```python
from build123d import *

# Parameters (mm, degrees)
ESQUISSE1_R             = 1
BOSS_EXTRU_1_DEPTH      = 6
ESQUISSE2_R             = 10
ESQUISSE2_R_2           = 2
ESQUISSE2_R_3           = 1.4
ESQUISSE2_R_4           = 1.5
ESQUISSE2_W             = 8
ESQUISSE2_H             = 55
ESQUISSE2_W_2           = 44
ESQUISSE2_W_3           = 40
ESQUISSE2_H_2           = 80
ENL_V_MAT_EXTRU_1_DEPTH = 6
ESQUISSE3_W             = 6
ESQUISSE3_H             = 10
ESQUISSE3_W_2           = 10
ESQUISSE3_H_2           = 6
ESQUISSE3_W_3           = 15
ENL_V_MAT_EXTRU_2_DEPTH = 6
ESQUISSE4_R             = 1.5
ENL_V_MAT_EXTRU_3_DEPTH = 6
ESQUISSE5_W             = 10
ESQUISSE5_H             = 6
ESQUISSE5_W_2           = 20
ENL_V_MAT_EXTRU_4_DEPTH = 6
ESQUISSE6_R             = 1.65
ESQUISSE6_R_2           = 1.5
ESQUISSE6_R_3           = 2
ENL_V_MAT_EXTRU_5_DEPTH = 6


with BuildPart() as part:
    # Esquisse1 → Boss.-Extru.1 (new body)
    with BuildSketch(Plane.XY):
        Polygon((-165, 96.73), (165, 96.73), (165, -18.27), (123, -109.022410436), (-123, -109.022410436), (-165, -18.27), align=None)
        with Locations((-23.6, -89.522410436)):
            Circle(ESQUISSE1_R, mode=Mode.SUBTRACT)
        with Locations((-23.6, -73.522410436)):
            Circle(ESQUISSE1_R, mode=Mode.SUBTRACT)
        with Locations((-39.6, -89.522410436)):
            Circle(ESQUISSE1_R, mode=Mode.SUBTRACT)
        with Locations((-39.6, -73.522410436)):
            Circle(ESQUISSE1_R, mode=Mode.SUBTRACT)
    extrude(amount=BOSS_EXTRU_1_DEPTH)

    # Esquisse2 → Enlèv. mat.-Extru.1 (cut)
    with BuildSketch(Plane.XY.offset(6)):
        with Locations((140, 76.73)):
            Circle(ESQUISSE2_R)
        with Locations((108, -89.022410436)):
            Circle(ESQUISSE2_R)
        with Locations((-140, 76.73)):
            Circle(ESQUISSE2_R)
        with Locations((-108, -89.022410436)):
            Circle(ESQUISSE2_R)
        with Locations((161, -16.022410436)):
            Circle(ESQUISSE2_R_2)
        with Locations((119, -105.022410436)):
            Circle(ESQUISSE2_R_2)
        with Locations((161, 92.73)):
            Circle(ESQUISSE2_R_2)
        with Locations((-161, 92.73)):
            Circle(ESQUISSE2_R_2)
        with Locations((-161, -16.022410436)):
            Circle(ESQUISSE2_R_2)
        with Locations((-119, -105.022410436)):
            Circle(ESQUISSE2_R_2)
        with Locations((125.27, 76.73)):
            Circle(ESQUISSE2_R_3)
        with Locations((110.27, 76.73)):
            Circle(ESQUISSE2_R_3)
        with Locations((114.7893454, -75.950391119)):
            Circle(ESQUISSE2_R_4)
        with Locations((121.703139086, -62.638762485)):
            Circle(ESQUISSE2_R_4)
        with Locations((-110.27, 76.73)):
            Circle(ESQUISSE2_R_3)
        with Locations((-125.27, 76.73)):
            Circle(ESQUISSE2_R_3)
        with Locations((-121.703139086, -62.638762485)):
            Circle(ESQUISSE2_R_4)
        with Locations((-114.7893454, -75.950391119)):
            Circle(ESQUISSE2_R_4)
        with Locations((-154, 28.477589564)):
            Rectangle(ESQUISSE2_W, ESQUISSE2_H)
        with Locations((-108, 28.477589564)):
            Rectangle(ESQUISSE2_W_2, ESQUISSE2_H)
        with Locations((108, 28.477589564)):
            Rectangle(ESQUISSE2_W_2, ESQUISSE2_H)
        with Locations((154, 28.477589564)):
            Rectangle(ESQUISSE2_W, ESQUISSE2_H)
        with Locations((69, -69.022410436)):
            Rectangle(ESQUISSE2_W_3, ESQUISSE2_H_2)
        with Locations((-69, -69.022410436)):
            Rectangle(ESQUISSE2_W_3, ESQUISSE2_H_2)
    extrude(amount=-ENL_V_MAT_EXTRU_1_DEPTH, mode=Mode.SUBTRACT)

    # Esquisse3 → Enlèv. mat.-Extru.2 (cut)
    with BuildSketch(Plane(origin=(0, 0, 0), x_dir=(-1, 0, 0), z_dir=(0, 0, -1))):
        with Locations((162, 1.73)):
            Rectangle(ESQUISSE3_W, ESQUISSE3_H)
        with Locations((162, 73.852589564)):
            Rectangle(ESQUISSE3_W, ESQUISSE3_H)
        with Locations((24.5, -106.022410436)):
            Rectangle(ESQUISSE3_W_2, ESQUISSE3_H_2)
        with Locations((-24.5, -106.022410436)):
            Rectangle(ESQUISSE3_W_2, ESQUISSE3_H_2)
        with Locations((-162, 73.852589564)):
            Rectangle(ESQUISSE3_W, ESQUISSE3_H)
        with Locations((-162, 1.73)):
            Rectangle(ESQUISSE3_W, ESQUISSE3_H)
        with Locations((107.5, 93.73)):
            Rectangle(ESQUISSE3_W_3, ESQUISSE3_H_2)
        with Locations((-42.5, 93.73)):
            Rectangle(ESQUISSE3_W_3, ESQUISSE3_H_2)
        with Locations((42.5, 93.73)):
            Rectangle(ESQUISSE3_W_3, ESQUISSE3_H_2)
        with Locations((-107.5, 93.73)):
            Rectangle(ESQUISSE3_W_3, ESQUISSE3_H_2)
    extrude(amount=-ENL_V_MAT_EXTRU_2_DEPTH, mode=Mode.SUBTRACT)

    # Esquisse4 → Enlèv. mat.-Extru.3 (cut)
    with BuildSketch(Plane(origin=(0, 0, 0), x_dir=(-1, 0, 0), z_dir=(0, 0, -1))):
        with Locations((162, -6.27)):
            Circle(ESQUISSE4_R)
        with Locations((0, -106.022410436)):
            Circle(ESQUISSE4_R)
        with Locations((162, 62.852589564)):
            Circle(ESQUISSE4_R)
        with Locations((0, 93.73)):
            Circle(ESQUISSE4_R)
        with Locations((-39.25, -106.022410436)):
            Circle(ESQUISSE4_R)
        with Locations((-14.75, -106.022410436)):
            Circle(ESQUISSE4_R)
        with Locations((14.75, -106.022410436)):
            Circle(ESQUISSE4_R)
        with Locations((39.25, -106.022410436)):
            Circle(ESQUISSE4_R)
        with Locations((150, 93.73)):
            Circle(ESQUISSE4_R)
        with Locations((125, 93.73)):
            Circle(ESQUISSE4_R)
        with Locations((90, 93.73)):
            Circle(ESQUISSE4_R)
        with Locations((-25, 93.73)):
            Circle(ESQUISSE4_R)
        with Locations((60, 93.73)):
            Circle(ESQUISSE4_R)
        with Locations((25, 93.73)):
            Circle(ESQUISSE4_R)
        with Locations((-60, 93.73)):
            Circle(ESQUISSE4_R)
        with Locations((-90, 93.73)):
            Circle(ESQUISSE4_R)
        with Locations((-125, 93.73)):
            Circle(ESQUISSE4_R)
        with Locations((-150, 93.73)):
            Circle(ESQUISSE4_R)
        with Locations((-162, 62.852589564)):
            Circle(ESQUISSE4_R)
        with Locations((-162, -6.27)):
            Circle(ESQUISSE4_R)
    extrude(amount=-ENL_V_MAT_EXTRU_3_DEPTH, mode=Mode.SUBTRACT)

    # Esquisse5 → Enlèv. mat.-Extru.4 (cut)
    with BuildSketch(Plane(origin=(0, 0, 0), x_dir=(-1, 0, 0), z_dir=(0, 0, -1))):
        with Locations((114, -35.022410436)):
            Rectangle(ESQUISSE5_W, ESQUISSE5_H)
        with Locations((24, -35.022410436)):
            Rectangle(ESQUISSE5_W_2, ESQUISSE5_H)
        with Locations((-24, -35.022410436)):
            Rectangle(ESQUISSE5_W_2, ESQUISSE5_H)
        with Locations((-114, -35.022410436)):
            Rectangle(ESQUISSE5_W, ESQUISSE5_H)
    extrude(amount=-ENL_V_MAT_EXTRU_4_DEPTH, mode=Mode.SUBTRACT)

    # Esquisse6 → Enlèv. mat.-Extru.5 (cut)
    with BuildSketch(Plane(origin=(0, 0, 0), x_dir=(-1, 0, 0), z_dir=(0, 0, -1))):
        with Locations((-140, 3.477589564)):
            Circle(ESQUISSE6_R)
        with Locations((-140, 53.477589564)):
            Circle(ESQUISSE6_R)
        with Locations((140, 53.477589564)):
            Circle(ESQUISSE6_R)
        with Locations((140, 3.477589564)):
            Circle(ESQUISSE6_R)
        with Locations((-39, -35.022410436)):
            Circle(ESQUISSE6_R_2)
        with Locations((9, -35.022410436)):
            Circle(ESQUISSE6_R_2)
        with Locations((39, -35.022410436)):
            Circle(ESQUISSE6_R_2)
        with Locations((-9, -35.022410436)):
            Circle(ESQUISSE6_R_2)
        with Locations((-78.5, 49.477589564)):
            Circle(ESQUISSE6_R_3)
        with Locations((-78.5, 7.477589564)):
            Circle(ESQUISSE6_R_3)
        with Locations((-60, 47.977589564)):
            Circle(ESQUISSE6_R_3)
        with Locations((-60, 8.977894939)):
            Circle(ESQUISSE6_R_3)
        with Locations((60, 8.977894939)):
            Circle(ESQUISSE6_R_3)
        with Locations((60, 47.977589564)):
            Circle(ESQUISSE6_R_3)
        with Locations((-50, 45.977589564)):
            Circle(ESQUISSE6_R_3)
        with Locations((50, 45.977589564)):
            Circle(ESQUISSE6_R_3)
        with Locations((50, 10.977589564)):
            Circle(ESQUISSE6_R_3)
        with Locations((-50, 10.977589564)):
            Circle(ESQUISSE6_R_3)
        with Locations((78.5, 7.477589564)):
            Circle(ESQUISSE6_R_3)
        with Locations((78.5, 49.477589564)):
            Circle(ESQUISSE6_R_3)
        with Locations((104.5, -27.222410436)):
            Circle(ESQUISSE6_R_2)
        with Locations((104.5, -50.222410436)):
            Circle(ESQUISSE6_R_2)
        with Locations((-104.5, -50.222410436)):
            Circle(ESQUISSE6_R_2)
        with Locations((-104.5, -27.222410436)):
            Circle(ESQUISSE6_R_2)
    extrude(amount=-ENL_V_MAT_EXTRU_5_DEPTH, mode=Mode.SUBTRACT)


solid = part.part
```
Work out the finished part from the listing and answer in its coordinate system (mm). A direction names the side the tool comes from. Round coordinates to 2 decimals unless told otherwise and drop trailing zeros. Write each loop counter-clockwise with the first axis right and the second up, starting at its lowest first coordinate (ties: lowest second). Pieces come first, ordered by that corner, then holes. Notation, with made-up numbers: (-3.75, 35) - (17.25, 35) arc R31 ccw to (17.25, 63) - close; hole circle Ø2 at (9.5, 84). An arc over 180 degrees is marked (long way). Return JSON: item names as keys, results as strings. Group by question number.
Q1. Find the intervals of material crossed by L1, parallel to X at y = 25, z = 3.65; L2, parallel to Y at x = 90, z = 3.75; L3, parallel to Y at x = 60, z = 3.95, in increasing order.
Q2. The mould has two halves that part along X. Classify faces 1 (the flat face through (-49, -70, 3)), 2 (the flat face through (39, -109.022, 3)), 3 (the flat face through (-24, -103.022, 3)): released by +X, released by -X, zero draft, split by the parting line, or undercut.
Q3. Each of these flat-tipped pins is pushed along its axis until it touches: pin 1 Ø3 at (y, z) = (-76.5, 3.5) entering from +X; pin 2 Ø3 at (y, z) = (-33.5, 3.5) entering from -X. Where does it stop, or does it pass through?
Q4. The part is cut by section B-B on z = 1.7. Count the separate pieces of the cut face and the enclosed holes in it, then the cut area to 3 significant figures.
Q5. For faces 4 (the flat face through (162, 68.853, 3)), 5 (the flat face through (35, 94, 3)), 6 (the flat face through (108, 0.978, 3)), 7 (the flat face through (-19.5, -106, 3)), determine the directions among +Z, -Z, +X, -X, +Y, -Y from which every point of the face is accessible in a straight line to the end or side of a thin tool.
Q6. The part is cut by section A-A on y = 22. Write down the section's boundary in (x, z), then the cut area to 3 significant figures.
Solved:
{
 "1": {"L1": "-165 to -158, -150 to -130, -86 to 86, 130 to 150, 158 to 165", "L2": "-109.02 to 0.98, 55.98 to 92.23, 95.23 to 96.73", "L3": "-29.02 to 6.98, 10.98 to 45.98, 49.98 to 92.23, 95.23 to 96.73"},
 "2": {"face 1": "undercut", "face 2": "zero draft", "face 3": "undercut"},
 "3": {"pin 1": "x = 138.75", "pin 2": "x = -158.65"},
 "4": {"separate pieces": "1", "enclosed holes": "74", "area": "49,100 mm²"},
 "5": {"face 4": "+Z, -Z, +X", "face 5": "+Z, -Z, +Y", "face 6": "+Z, -Z", "face 7": "+Z, -Z, -Y"},
 "6": {"outline": "(-165, 0) - (-158, 0) - (-158, 6) - (-165, 6) - close; (-150, 0) - (-130, 0) - (-130, 6) - (-150, 6) - close; (-86, 0) - (86, 0) - (86, 6) - (-86, 6) - close; (130, 0) - (150, 0) - (150, 6) - (130, 6) - close; (158, 0) - (165, 0) - (165, 6) - (158, 6) - close", "area": "1,360 mm²"}
}
